Read the model definition and answer for the solid it produces. Units are mm, in the model's axes. A direction names the side the tool comes from. Give positions to 0.01 mm unless a question says otherwise; leave off trailing zeros. Write each loop counter-clockwise with the first axis right and the second up, starting at its lowest first coordinate (ties: lowest second). Pieces come first, ordered by that corner, then holes. Notation, with made-up numbers: (-11.5, -38.5) -> (5.5, -38.5) arc R33 ccw to (5.5, -1.5) -> close; hole circle Ø3 at (52, 61.25). An arc over 180 degrees is marked (long way). Put each result on its own line as item: value. Start each with the question number.
from build123d import *

# Parameters (mm, degrees)
SKETCH_W        = 44
SKETCH_H        = 11
PAD_DEPTH       = 40
SKETCH001_W     = 42
SKETCH001_H     = 9
POCKET_DEPTH    = 39.001
SKETCH002_R     = 12.5
POCKET001_DEPTH = 1
FILLET_R        = 1
FILLET001_R     = 0.5


with BuildPart() as part:
    # Sketch → Pad (new body)
    with BuildSketch(Plane.XY):
        with Locations((22, 5.5)):
            Rectangle(SKETCH_W, SKETCH_H)
    extrude(amount=PAD_DEPTH)

    # Sketch001 → Pocket (cut, through all)
    with BuildSketch(Plane.XY.offset(1)):
        with Locations((22, 5.5)):
            Rectangle(SKETCH001_W, SKETCH001_H)
    extrude(amount=POCKET_DEPTH, mode=Mode.SUBTRACT)

    # Sketch002 (on Face1 of Pocket) → Pocket001 (cut)
    with BuildSketch(Plane.XZ):
        with Locations((21, 40)):
            Circle(SKETCH002_R)
    extrude(amount=-POCKET001_DEPTH, mode=Mode.SUBTRACT)

    # Fillet
    fillet_edges = [part.edges().sort_by_distance(p)[0] for p in [
        (0, 0, 20),
        (0, 11, 20),
        (44, 0, 20),
        (44, 11, 20),
        (44, 5.5, 0),
        (22, 0, 0),
        (22, 11, 0),
        (0, 5.5, 0),
    ]]
    fillet(fillet_edges, radius=FILLET_R)

    # Fillet001
    fillet001_edges = [part.edges().sort_by_distance(p)[0] for p in [
        (21, 0, 27.5),
        (4.75, 0, 40),
        (0, 5.5, 40),
        (0.292893, 0.292893, 40),
        (0.292893, 10.707107, 40),
        (22, 11, 40),
        (44, 5.5, 40),
        (43.707107, 10.707107, 40),
        (43.707107, 0.292893, 40),
        (38.25, 0, 40),
    ]]
    fillet(fillet001_edges, radius=FILLET001_R)


solid = part.part
1) A cutting plane is placed at B-B on x = 39.5. Give the vertices of the cut face in (y, z).
2) For faces 5 (the face through (20.725, 0.746, 27.503)), 6 (the face through (22, 6, 0)), 7 (the face through (22, 1, 16)), determine the directions among +Z, -Z, +X, -X, +Y, -Y from which every point of the face is accessible in a straight line to the end or side of a thin tool.
3) A cutting plane is placed at C-C on y = 8.5. Give the vertices of the cut face in (x, z).
4) A cutting plane is placed at A-A on z = 16. Give the vertices of the cut face in (x, y), and give its area (3 significant figures).
5) This flat-tipped pin is pushed along its axis until it touches: pin 1 Ø2.5 at (x, y) = (32.5, 6) entering from +Z. Where does it stop, or does it pass through?
6) For a pull along X with two mould halves and no side action, classify faces 1 (the face through (22, 0, 16)), 2 (the face through (0, 5, 20)), 3 (the face through (44, 5, 20)), 4 (the face through (43, 5, 20)) as pulls with the +X half, pulls with the -X half, needs draft (parallel to the pull), parting line crosses it, or undercut.
7) Straight lines are drawn through the part: line 1 (Y direction, x = 25.5, z = 8.5); line 2 (X direction, y = 2.75, z = 2); line 3 (Z direction, x = 2, y = 5.75). For each, find the intervals that lie inside material, in ascending order. Write a range as [from, to].
Results found:
1. outline: (0, 1) arc R1 ccw to (1, 0) -> (10, 0) arc R1 ccw to (11, 1) -> (11, 39.5) arc R0.5 ccw to (10.5, 40) -> (10, 40) -> (10, 1) -> (1, 1) -> (1, 40) -> (0.5, 40) arc R0.5 ccw to (0, 39.5) -> close
2. face 5: +Z, -Y
2. face 6: -Z, +X, -X, +Y, -Y
2. face 7: +Z
3. outline: (0, 1) arc R1 ccw to (1, 0) -> (43, 0) arc R1 ccw to (44, 1) -> (44, 39.5) arc R0.5 ccw to (43.5, 40) -> (43, 40) -> (43, 1) -> (1, 1) -> (1, 40) -> (0.5, 40) arc R0.5 ccw to (0, 39.5) -> close
4. outline: (0, 1) arc R1 ccw to (1, 0) -> (43, 0) arc R1 ccw to (44, 1) -> (44, 10) arc R1 ccw to (43, 11) -> (1, 11) arc R1 ccw to (0, 10) -> close; hole (1, 1) -> (43, 1) -> (43, 10) -> (1, 10) -> close
4. area: 105 mm²
5. pin 1: stops at z = 1
6. face 1: needs draft
6. face 2: pulls with the -X half
6. face 3: pulls with the +X half
6. face 4: undercut
7. line 1: y = [0, 1], [10, 11]
7. line 2: x = [0, 1], [43, 44]
7. line 3: z = [0, 1]
